Work out the finished part from the listing and answer in its coordinate system (mm). A direction names the side the tool comes from. Round coordinates to 2 decimals unless told otherwise and drop trailing zeros. Loops run counter-clockwise (first coordinate to the right, second up) from the corner with the lowest first, then second, coordinate; pieces in that order, holes last. Notation, with made-up numbers: (49, 28.25) - (104, 28.25) arc R24 ccw to (104, 50.25) - close; hole circle Ø3 at (88.5, 56). An arc over 180 degrees is marked (long way). Answer as CSV lines item,"result". Start each with the question number.
Q1. Section A-A on x = 22.5 is taken. Write down the section's boundary in (y, z), then the cut area to 3 significant figures.
Q2. Straight lines are drawn through the part: L1, parallel to Y at x = 54.5, z = 0; L2, parallel to Z at x = 65.35, y = 0; L3, parallel to X at y = -16, z = 4. For each, find the intervals that lie inside material, in ascending order. Write a range as [from, to].
Q3. Each of these flat-tipped pins is pushed along its axis until it touches: pin 1 Ø6 at (x, y) = (60.5, 15.5) entering from -Z; pin 2 Ø8 at (x, z) = (51, -11) entering from -Y; pin 3 Ø8 at (x, z) = (59, 20) entering from +Y; pin 4 Ø17 at (y, z) = (0, 0) entering from -X. Where does it stop, or does it pass through?
Q4. The mould has two halves that part along Y. Classify faces 1 (the face through (72.93, -29.47, 0.65)), 2 (the face through (77.812, 15.691, -24.611)), 3 (the face through (30.008, 22.637, -5.027)): +Y half, -Y half, draft (parallel to the pull), parting line (faces both ways), or undercut.
Q5. For faces 4 (the face through (72.93, 0.65, 29.47)), 5 (the face through (72.93, 29.47, -0.65)), 6 (the face through (78, -13.3, -12.5)), determine the directions among +Z, -Z, +X, -X, +Y, -Y from which every point of the face is accessible in a straight line to the end or side of a thin tool.
Autodesk Inventor part; units mm, degrees
ref_plane "РабПлоскость1" through (65.5, 32, 0) normal (0, 1, 0) x (-1, 0, 0)
ref_plane "YZ Plane" through (0, 0, 0) normal (1, 0, 0) x (0, 1, 0)
ref_plane "XY Plane" through (0, 0, 0) normal (0, 0, 1) x (1, 0, 0)
sketch "Эскиз1" plane through (0, 0, 0) normal (0, 0, 1) x (1, 0, 0)
  line L0 (0, 0) -> (100, 0)
  line L1 (0, 20) -> (0, 32)
  line L2 (0, 32) -> (13, 32)
  line L3 (13, 32) -> (13, 30)
  line L4 (13, 30) -> (53, 30)
  line L5 (53, 30) -> (53, 32)
  line L6 (53, 32) -> (78, 32)
  line L7 (78, 32) -> (78, 18)
  line L8 (78, 18) -> (100, 18)
  line L9 (100, 18) -> (100, 10.5)
  line L10 (100, 10.5) -> (70, 10.5)
  line L11 (70, 10.5) -> (70, 19)
  line L12 (70, 19) -> (64, 19)
  line L13 (64, 19) -> (64, 24.6)
  line L14 (0, 20) -> (56, 20)
  line L15 (56, 20) -> (60.8828, 24.8828)
  line L16 (61.1657, 25) -> (63.6, 25)
  arc A0 (61.1657, 25) -> (60.8828, 24.8828) centre (61.1657, 24.6) ccw
  arc A1 (64, 24.6) -> (63.6, 25) centre (63.6, 24.6) ccw
  point P0 (64, 25)
  point P1 (61, 25)
  dimension "d2" = 100
  dimension "d3" = 40
  dimension "d4" = 25
  dimension "d5" = 22
  dimension "d6" = 21
  dimension "d7" = 36
  dimension "d11" = 38
  dimension "d12" = 6
  dimension "d13" = 64
  dimension "d14" = 64
  dimension "d15" = 60
  dimension "d16" = 45
  dimension "d18" = 3
  dimension "d19" = 0.4
  dimension "d20" = 50
  dimension "d21" = 40
revolve "Вращение1" add sketch "Эскиз1" angle 360 about axis through (0, 0, 0) along (1, 0, 0)
sketch "Эскиз2" plane through (0, 0, 0) normal (-1, 0, 0) x (0, 0, 1)
  circle A0 centre (0, 0) radius 32
hole "Отверстие1" at (0, 0, 0) direction (1, 0, 0) diameter 46.376 depth 61
ref_plane "РабПлоскость1" through (65.5, 32, 0) normal (0, 1, 0) x (-1, 0, 0)
sketch "Эскиз3" plane through (65.5, 32, 0) normal (0, 1, 0) x (-1, 0, 0)
  line L0 (-12.5, 32) -> (-12.5, -32)
  point P0 (65.5, 0)
  point P1 (-4.5, 0)
  dimension "d29" = 8
hole "Отверстие2" at (70, 32, 0) direction (0, -1, 0) diameter 6 depth 5 tip angle 118
pattern_circular "Круговой массив1" count 4 over 360 about axis through (65.5, 0, 0) along (1, 0, 0) of "Отверстие2"
chamfer "Фаска1" distance 3 angle 45 1 edges at (78, -32, 0)
chamfer "Фаска2" distance 1 angle 45 1 edges at (0, -32, 0)
properties part number "05.01.006" material "Чугун, серый"
Findings:
1,outline,"circle Ø60 at (0, 0); hole circle Ø46.38 at (0, 0)"
1,area,"1,140 mm^2"
2,L1,"y = [-32, -23.19], [23.19, 32]"
2,L2,"z = [-32, -19], [19, 32]"
2,L3,"x = [70, 100]"
3,pin 1,"stops at z = -29.46"
3,pin 2,"stops at y = -31.1"
3,pin 3,"stops at y = 27.71"
3,pin 4,"passes through"
4,face 1,"draft"
4,face 2,"parting line"
4,face 3,"undercut"
5,face 4,"+Z"
5,face 5,"+Y"
5,face 6,"+X"
